```python
from build123d import *

# Parameters (mm, degrees)
F0_R     = 16.8656
F1_DEPTH = 6.35


with BuildPart() as f1:
    # F0 (on Top) → F1 (new body)
    with BuildSketch(Plane.XY):
        with BuildLine():
            ThreePointArc((69.431615, -39.890337), (71.634026, -36.594196), (72.40741, -32.706132))
            Line((72.40741, -32.706132), (72.40741, -18.516952))
            ThreePointArc((72.40741, -18.516952), (71.634026, -14.628888), (69.431615, -11.332747))
            Line((69.431615, -11.332747), (61.286205, -3.187337))
            ThreePointArc((61.286205, -3.187337), (57.990064, -0.984926), (54.102, -0.211542))
            Line((54.102, -0.211542), (21.914013, -0.211542))
            ThreePointArc((21.914013, -0.211542), (16.111142, -1.359548), (11.182513, -4.630613))
            Line((11.182513, -4.630613), (4.930193, -10.831261))
            ThreePointArc((4.930193, -10.831261), (1.482689, -15.956217), (0.27141, -22.012888))
            Line((0.27141, -22.012888), (0.27141, -29.210196))
            ThreePointArc((0.27141, -29.210196), (1.482689, -35.266867), (4.930193, -40.391823))
            Line((4.930193, -40.391823), (11.182513, -46.592471))
            ThreePointArc((11.182513, -46.592471), (16.111142, -49.863535), (21.914013, -51.011542))
            Line((21.914013, -51.011542), (54.102, -51.011542))
            ThreePointArc((54.102, -51.011542), (57.990064, -50.238158), (61.286205, -48.035747))
            Line((61.286205, -48.035747), (69.431615, -39.890337))
        make_face()
        with BuildLine():
            Line((27.85581, -15.451542), (27.85581, -35.771542))
            ThreePointArc((27.85581, -35.771542), (25.549569, -41.339301), (19.98181, -43.645542))
            ThreePointArc((19.98181, -43.645542), (16.96856, -43.046169), (14.414051, -41.339301))
            Line((14.414051, -41.339301), (7.403651, -34.328901))
            ThreePointArc((7.403651, -34.328901), (5.696782, -31.774391), (5.09741, -28.761142))
            Line((5.09741, -28.761142), (5.09741, -22.461942))
            ThreePointArc((5.09741, -22.461942), (5.696782, -19.448693), (7.403651, -16.894183))
            Line((7.403651, -16.894183), (14.414051, -9.883783))
            ThreePointArc((14.414051, -9.883783), (22.995059, -8.176915), (27.85581, -15.451542))
        make_face(mode=Mode.SUBTRACT)
        with Locations((50.43641, -25.611542)):
            Circle(F0_R, mode=Mode.SUBTRACT)
    extrude(amount=F1_DEPTH)


solid = f1.part
```
Model file for the job. Use its own axes, mm. A direction names the side the tool comes from. Coordinates: 2 decimals unless noted, no trailing zeros. Loops run counter-clockwise (first coordinate to the right, second up) from the corner with the lowest first, then second, coordinate; pieces in that order, holes last. Notation, with made-up numbers: M 13.5,-38.75 L 44.5,-38.75 A17 cw 44.5,-28.75 Z; hole C -18.5,-10 d6. An arc over 180 degrees is marked long. Use CSV: the item, a comma, the result in double quotes. Start each with the question number.
1. Band-saw the part on D-D, the plane x = 38. List the corners of the cut face in (y, z), then the cut area to 3 significant figures.
2. Band-saw the part on B-B, the plane y = -36.5. List the corners of the cut face in (x, z).
3. Tool access for faces 1 (the flat face through (0.271, -26, 3)), 2 (the cylindrical face through (22.875, -8.128, 3.131)): list every direction of +Z, -Z, +X, -X, +Y, -Y with a clear straight run to the whole face (end or side of a thin tool).
4. Flat gauge pins, fed straight in: pin 1 (1.5 mm diameter, centred on y = -12, z = 2.5, fed in from -X); pin 2 (2 mm diameter, centred on y = -7, z = 3, fed in from -X). Where does each tip first touch, or does it go through?
5. Two-plate mould, pull along Y, no slides. Class faces 3 (the flat face through (65.4, -7.3, 3.1)), 4 (the cylindrical face through (71.61, -36.65, 3.13)), 5 (the flat face through (10.9, -13.4, 3.1)): pulls with the +Y half, pulls with the -Y half, needs draft (parallel to the pull), parting line crosses it, or undercut.
6. Probe probe 1 along Y at (x, z) = (50, 5); probe 2 along X at (y, z) = (-10.5, 0.75); probe 3 along X at (y, z) = (-19, 0.75). List the from-to ranges inside material, lowest first. Write a range as [from, to].
7. Band-saw the part on A-A, the plane x = 26.5. List the corners of the cut face in (y, z), then the cut area to 3 significant figures.
8. Band-saw the part on C-C, the plane z = 3.25. List the corners of the cut face in (x, y).
Entries:
1,outline,"M -51.01,0 L -37,0 L -37,6.35 L -51.01,6.35 Z; M -14.22,0 L -0.21,0 L -0.21,6.35 L -14.22,6.35 Z"
1,area,"178 mm2"
2,outline,"M 2.06,0 L 9.57,0 L 9.57,6.35 L 2.06,6.35 Z; M 27.82,0 L 37.56,0 L 37.56,6.35 L 27.82,6.35 Z; M 63.32,0 L 71.67,0 L 71.67,6.35 L 63.32,6.35 Z"
3,face 1,"+Z, -Z, -X, +Y, -Y"
3,face 2,"+Z, -Z"
4,pin 1,"stops at x = 3.28"
4,pin 2,"stops at x = 7.79"
5,face 3,"pulls with the +Y half"
5,face 4,"pulls with the -Y half"
5,face 5,"undercut"
6,probe 1,"y = [-51.01, -42.47], [-8.75, -0.21]"
6,probe 2,"x = [5.26, 13.8], [26.1, 42.95], [57.93, 68.6]"
6,probe 3,"x = [0.56, 5.9], [27.86, 34.92], [65.95, 72.41]"
7,outline,"M -51.01,0 L -40.19,0 L -40.19,6.35 L -51.01,6.35 Z; M -11.03,0 L -0.21,0 L -0.21,6.35 L -11.03,6.35 Z"
7,area,"137 mm2"
8,outline,"M 0.27,-29.21 A15.75 ccw 4.93,-40.39 L 11.18,-46.59 A15.24 ccw 21.91,-51.01 L 54.1,-51.01 A10.16 ccw 61.29,-48.04 L 69.43,-39.89 A10.16 ccw 72.41,-32.71 L 72.41,-18.52 A10.16 ccw 69.43,-11.33 L 61.29,-3.19 A10.16 ccw 54.1,-0.21 L 21.91,-0.21 A15.24 ccw 11.18,-4.63 L 4.93,-10.83 A15.75 ccw 0.27,-22.01 Z; hole M 5.1,-28.76 A7.87 ccw 7.4,-34.33 L 14.41,-41.34 A7.87 ccw 19.98,-43.65 A7.87 ccw 27.86,-35.77 L 27.86,-15.45 A7.87 ccw 14.41,-9.88 L 7.4,-16.89 A7.87 ccw 5.1,-22.46 Z; hole C 50.44,-25.61 d33.73"
